Could you check a few things on this model? Use its own coordinates, in mm. Face numbers are marked on the shaded views. A direction names the side the tool comes from. Coordinates: 2 decimals unless noted, no trailing zeros. Write each loop counter-clockwise with the first axis right and the second up, starting at its lowest first coordinate (ties: lowest second). Pieces come first, ordered by that corner, then holes.
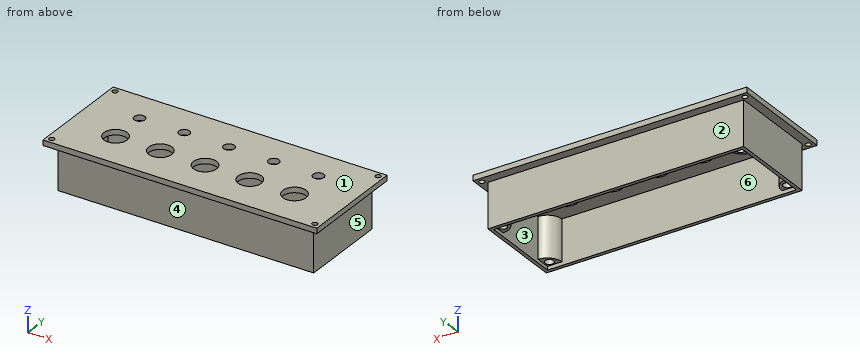
```python
from build123d import *

# Parameters (mm, degrees)
SKETCH_W                      = 153
SKETCH_H                      = 60
PAD_DEPTH                     = 3
SKETCH002_W                   = 143
SKETCH002_H                   = 50
SKETCH002_W_2                 = 139
SKETCH002_H_2                 = 46
PAD001_DEPTH                  = 25
SKETCH003_R                   = 1.5
POCKET_DEPTH                  = 3.001
PAD002_DEPTH                  = 23
PAD002_MIRRORED_2_DEPTH       = 23
SKETCH005_R                   = 2.4
POCKET001_DEPTH               = 10
SKETCH005_MIRRORED002_2_R     = 2.4
POCKET001_MIRRORED002_2_DEPTH = 10
SKETCH006_R                   = 6.5
SKETCH006_R_2                 = 3
POCKET002_DEPTH               = 28.001


with BuildPart() as part:
    # Sketch → Pad (new body)
    with BuildSketch(Plane.XY):
        Rectangle(SKETCH_W, SKETCH_H)
    extrude(amount=PAD_DEPTH)

    # Sketch002 (on Face5 of Pad) → Pad001 (join)
    with BuildSketch(Plane(origin=(0, 0, 0), x_dir=(1, 0, 0), z_dir=(0, 0, -1))):
        Rectangle(SKETCH002_W, SKETCH002_H)
        Rectangle(SKETCH002_W_2, SKETCH002_H_2, mode=Mode.SUBTRACT)
    extrude(amount=PAD001_DEPTH)

    # Sketch003 (on Face4 of Pad001) → Pocket (cut, through all)
    with BuildSketch(Plane(origin=(0, 0, 0), x_dir=(1, 0, 0), z_dir=(0, 0, -1))):
        with Locations((-73.5, 27)):
            Circle(SKETCH003_R)
        with Locations((-73.5, -27)):
            Circle(SKETCH003_R)
        with Locations((73.5, -27)):
            Circle(SKETCH003_R)
        with Locations((73.5, 27)):
            Circle(SKETCH003_R)
    extrude(amount=-POCKET_DEPTH, mode=Mode.SUBTRACT)

    # Sketch004 (on Face20 of Pocket) → Pad002 (join)
    with BuildSketch(Plane(origin=(0, 0, 0), x_dir=(1, 0, 0), z_dir=(0, 0, -1))):
        with BuildLine():
            Line((-69.5, 23), (-61.5, 23))
            ThreePointArc((-69.5, 15), (-63.843146, 17.343146), (-61.5, 23))
            Line((-69.5, 23), (-69.5, 15))
        make_face()
    pad002 = extrude(amount=PAD002_DEPTH)

    # Sketch004 Mirrored 2 → Pad002 Mirrored 2 (add)
    with BuildSketch(Plane(origin=(0, 0, 0), x_dir=(-1, 0, 0), z_dir=(0, 0, 1))):
        with BuildLine():
            Line((-69.5, 23), (-61.5, 23))
            ThreePointArc((-69.5, 15), (-63.843146, 17.343146), (-61.5, 23))
            Line((-69.5, 23), (-69.5, 15))
        make_face()
    pad002_mirrored_2 = extrude(amount=-PAD002_MIRRORED_2_DEPTH)

    # Mirrored001: Pad002, Pad002 Mirrored 2 across Sketch004 H_Axis
    add(pad002.mirror(Plane(origin=(0, 0, 0), x_dir=(0, 0, -1), z_dir=(0, -1, 0))))
    add(pad002_mirrored_2.mirror(Plane(origin=(0, 0, 0), x_dir=(0, 0, -1), z_dir=(0, -1, 0))))

    # Sketch005 (on Face20 of MultiTransform) → Pocket001 (cut)
    with BuildSketch(Plane(origin=(0, 0, -23), x_dir=(1, 0, 0), z_dir=(0, 0, -1))):
        with Locations((-66.5, 20)):
            Circle(SKETCH005_R)
    pocket001 = extrude(amount=-POCKET001_DEPTH, mode=Mode.SUBTRACT)

    # Sketch005 Mirrored002 2 → Pocket001 Mirrored002 2 (cut)
    with BuildSketch(Plane(origin=(0, 0, -23), x_dir=(-1, 0, 0), z_dir=(0, 0, 1))):
        with Locations((-66.5, 20)):
            Circle(SKETCH005_MIRRORED002_2_R)
    pocket001_mirrored002_2 = extrude(amount=POCKET001_MIRRORED002_2_DEPTH, mode=Mode.SUBTRACT)

    # Mirrored003: Pocket001, Pocket001 Mirrored002 2 across Sketch005 H_Axis
    add(pocket001.mirror(Plane(origin=(0, 0, -23), x_dir=(0, 0, -1), z_dir=(0, -1, 0))), mode=Mode.SUBTRACT)
    add(pocket001_mirrored002_2.mirror(Plane(origin=(0, 0, -23), x_dir=(0, 0, -1), z_dir=(0, -1, 0))), mode=Mode.SUBTRACT)

    # Sketch006 (on Face5 of MultiTransform001) → Pocket002 (cut, through all)
    with BuildSketch(Plane.XY.offset(3)):
        with Locations((-50, -8.5)):
            Circle(SKETCH006_R)
        with Locations((-25, -8.5)):
            Circle(SKETCH006_R)
        with Locations((0, -8.5)):
            Circle(SKETCH006_R)
        with Locations((25, -8.5)):
            Circle(SKETCH006_R)
        with Locations((50, -8.5)):
            Circle(SKETCH006_R)
        with Locations((-50, 12)):
            Circle(SKETCH006_R_2)
        with Locations((-25, 12)):
            Circle(SKETCH006_R_2)
        with Locations((0, 12)):
            Circle(SKETCH006_R_2)
        with Locations((25, 12)):
            Circle(SKETCH006_R_2)
        with Locations((50, 12)):
            Circle(SKETCH006_R_2)
    extrude(amount=-POCKET002_DEPTH, mode=Mode.SUBTRACT)


solid = part.part
```
Item 1: I want a section at A-A, the plane y = 12. Count the separate pieces of the cut face and the enclosed holes in it, then the cut area to 3 significant figures.
Item 2: Will these pins go through, and if not, where does the flat tip stop? pin 1 Ø3.5 at (x, y) = (-50, 12) entering from +Z; pin 2 Ø12.5 at (y, z) = (9, -11.5) entering from +X; pin 3 Ø1.4 at (x, y) = (-66.5, 19) entering from -Z; pin 4 Ø1.5 at (x, y) = (-0.5, 4) entering from -Z.
Item 3: If I drill on line 1 along Y through (x, z) = (-50, 1.05); line 2 along Y through (x, z) = (73.5, 1.4); line 3 along Y through (x, z) = (-30, -18.5), over which ranges is the centre line in solid material (lowest first)?
Item 4: If we mould it in two halves opening along Y, with no side actions, what happens to the marked faces 1, 2 and 3? For each: released by +Y, released by -Y, zero draft, split by the parting line, or undercut.
Item 5: I want a section at C-C, the plane x = -50. List the corners of the cut face in (y, z) for me, then the cut area to 3 significant figures.
Item 6: I want a section at B-B, the plane z = -20.5. List the corners of the cut face in (x, y) for me, then the cut area to 3 significant figures.
Item 7: I want a section at D-D, the plane y = 6. List the corners of the cut face in (x, z) for me, then the cut area to 3 significant figures.
Item 8: Which directions (+Z, -Z, +X, -X, +Y, -Y) give clear straight access to the entire face, cutting with the end or side of a thin tool? Please do the marked faces 4, 5 and 6.
Taken from the geometry:
1. separate pieces: 6
1. enclosed holes: 0
1. area: 469 mm2
2. pin 1: passes through
2. pin 2: stops at x = 71.5
2. pin 3: stops at z = -13
2. pin 4: stops at z = 0
3. line 1: y = -30 to -15, -2 to 9, 15 to 30
3. line 2: y = -30 to -28.5, -25.5 to 25.5, 28.5 to 30
3. line 3: y = -25 to -23, 23 to 25
4. face 1: zero draft
4. face 2: released by +Y
4. face 3: undercut
5. outline: (-30, 0) - (-25, 0) - (-25, -25) - (-23, -25) - (-23, 0) - (-15, 0) - (-15, 3) - (-30, 3) - close; (-2, 0) - (9, 0) - (9, 3) - (-2, 3) - close; (15, 0) - (23, 0) - (23, -25) - (25, -25) - (25, 0) - (30, 0) - (30, 3) - (15, 3) - close
5. area: 223 mm2
6. outline: (-71.5, -25) - (71.5, -25) - (71.5, 25) - (-71.5, 25) - close; hole (-69.5, -15) arc R8 cw to (-61.5, -23) - (61.5, -23) arc R8 cw to (69.5, -15) - (69.5, 15) arc R8 cw to (61.5, 23) - (-61.5, 23) arc R8 cw to (-69.5, 15) - close; hole circle Ø4.8 at (-66.5, -20); hole circle Ø4.8 at (-66.5, 20); hole circle Ø4.8 at (66.5, -20); hole circle Ø4.8 at (66.5, 20)
6. area: 885 mm2
7. outline: (-76.5, 0) - (-71.5, 0) - (-71.5, -25) - (-69.5, -25) - (-69.5, 0) - (69.5, 0) - (69.5, -25) - (71.5, -25) - (71.5, 0) - (76.5, 0) - (76.5, 3) - (-76.5, 3) - close
7. area: 559 mm2
8. face 4: -Z, +X, -X, -Y
8. face 5: -Z, +X, +Y, -Y
8. face 6: -Z
